Part model, mm, in its own coordinate system. Round coordinates to 2 decimals unless told otherwise and drop trailing zeros. Write each loop counter-clockwise with the first axis right and the second up, starting at its lowest first coordinate (ties: lowest second). Pieces come first, ordered by that corner, then holes.
```python
from build123d import *

# Parameters (mm, degrees)
SKETCH_1_W          = 231
SKETCH_1_H          = 70
SKETCH_1_R          = 2.5
EXTRUDE_1_DEPTH     = 3
SKETCH_4_R          = 1.5
CUT_EXTRUDE_1_DEPTH = 10


with BuildPart() as part:
    # 草图1 → 凸台-拉伸1 (new body)
    with BuildSketch(Plane.XY):
        Rectangle(SKETCH_1_W, SKETCH_1_H)
        with Locations((-107, 27.5)):
            Circle(SKETCH_1_R, mode=Mode.SUBTRACT)
        with Locations(Location((-107, -27.5, 0), (0, 0, 180))):
            Circle(SKETCH_1_R, mode=Mode.SUBTRACT)
        with Locations((107, -27.5)):
            Circle(SKETCH_1_R, mode=Mode.SUBTRACT)
        with Locations(Location((107, 27.5, 0), (0, 0, 180))):
            Circle(SKETCH_1_R, mode=Mode.SUBTRACT)
    extrude(amount=EXTRUDE_1_DEPTH)

    # 草图4 → 切除-拉伸1 (cut)
    with BuildSketch(Plane.XY.offset(3)):
        with Locations((-106.677486576, -19)):
            Circle(SKETCH_4_R)
    cut_extrude_1 = extrude(amount=-CUT_EXTRUDE_1_DEPTH, mode=Mode.SUBTRACT)

    # 镜向1: 切除-拉伸1 across plane
    add(cut_extrude_1.mirror(Plane(origin=(0, 0, 0), x_dir=(0, 0, 1), z_dir=(1, 0, 0))), mode=Mode.SUBTRACT)


solid = part.part
```
Q1. Cut at A-A on y = -27.5. Write the cut outline in (x, z).
Values follow:
outline: (-115.5, 0) - (-109.5, 0) - (-109.5, 3) - (-115.5, 3) - close; (-104.5, 0) - (104.5, 0) - (104.5, 3) - (-104.5, 3) - close; (109.5, 0) - (115.5, 0) - (115.5, 3) - (109.5, 3) - close
Q2. Drop flat-ended pins along their axis: pin 1 (8 mm diameter, centred on x = -107, y = -27.5, fed in from +Z); pin 2 (2.5 mm diameter, centred on x = -106.68, y = -19, fed in from +Z). Give the stop position or say it passes through.
Values follow:
pin 1: stops at z = 3
pin 2: passes through
Q3. Wall check: L1, parallel to Y at x = 107, z = 1.1. Give the ranges that are in metal, low to high.
Values follow:
L1: y = -35 to -30, -25 to -20.46, -17.54 to 25, 30 to 35
Q4. Mould opens along X. For faces 1 (the cylindrical face through (109.385, -26.749, 1.479)), 2 (the flat face through (-2, 0, 3)) say: +X half, -X half, draft (parallel to the pull), parting line (faces both ways), or undercut.
Values follow:
face 1: undercut
face 2: draft
